Source: three-view drawing plus pictorial views. Frame: mm from the lowest corner of the part. A direction names the side the tool comes from. Give positions to 0.01 mm unless a question says otherwise; leave off trailing zeros. Loops run counter-clockwise (first coordinate to the right, second up) from the corner with the lowest first, then second, coordinate; pieces in that order, holes last. Notation, with made-up numbers: (74.25, 34) - (119.25, 34) arc R30 cw to (119.25, 73) - close; hole circle Ø9 at (73, 42.25). An arc over 180 degrees is marked (long way). Put each result on its own line as item: value.
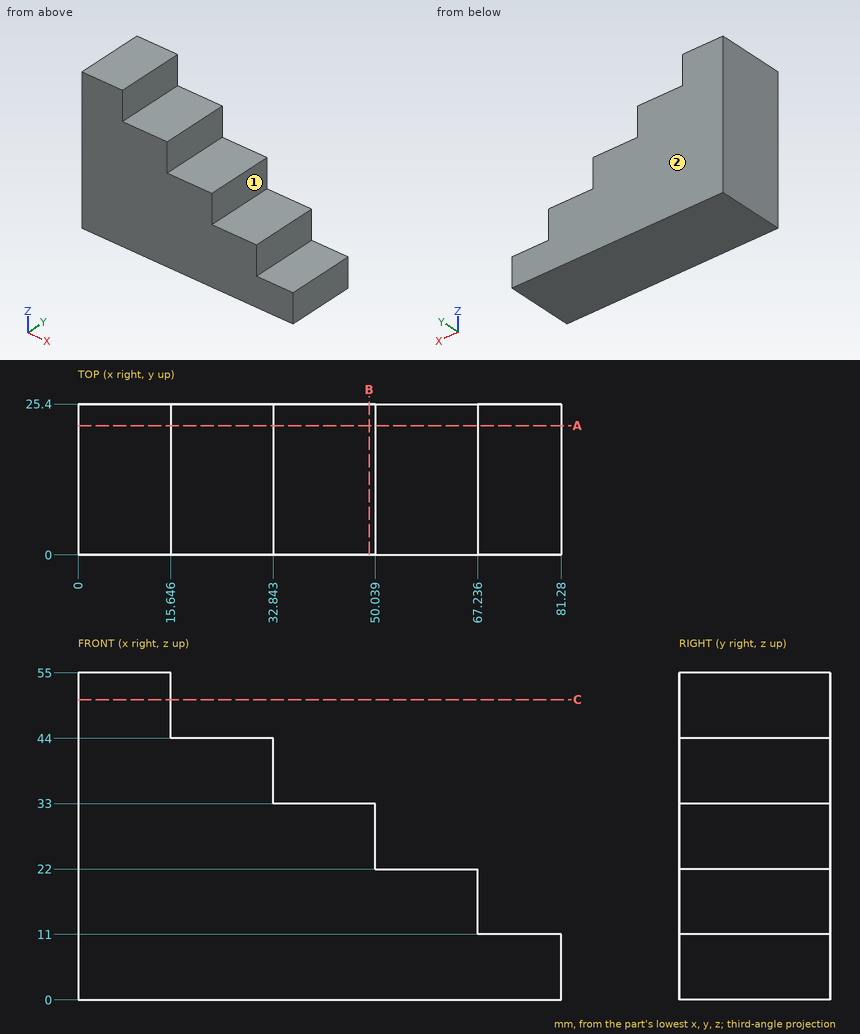
1) Section query A-A, the plane y = 21.75. Output: boundary loops of the cut face in (x, z).
Check result:
outline: (0, 0) - (81.28, 0) - (81.28, 11) - (67.24, 11) - (67.24, 22) - (50.04, 22) - (50.04, 33) - (32.84, 33) - (32.84, 44) - (15.65, 44) - (15.65, 55) - (0, 55) - close
2) Section query B-B, the plane x = 49. Output: boundary loops of the cut face in (y, z).
Check result:
outline: (0, 0) - (25.4, 0) - (25.4, 33) - (0, 33) - close
3) Section query C-C, the plane z = 50.5. Output: boundary loops of the cut face in (x, y).
Check result:
outline: (0, 0) - (15.65, 0) - (15.65, 25.4) - (0, 25.4) - close
4) Pin query (flat end, axial travel): P1, Ø6, axis at y = 8, z = 44, coming from the +X side; P2, Ø11, axis at x = 77.5, y = 12, coming from the +Z side; P3, Ø4, axis at x = 23, y = 14.5, coming from the +Z side. Return the tip coordinate at first contact, or that it passes through.
Check result:
P1: x = 32.84
P2: z = 11
P3: z = 44
5) Access query for the marked faces 1 and 2. Directions: +Z, -Z, +X, -X, +Y, -Y. A direction counts if a zero-diameter tool reaches every point of the face in a straight line with its end or side. Return the directions, or none.
Check result:
face 1: +Z, +X, +Y, -Y
face 2: +Z, -Z, +X, -X, +Y
6) Material intervals for line 1 along Z through (x, y) = (64, 3); line 2 along X through (y, z) = (21, 22.5); line 3 along X through (y, z) = (21.25, 20), sorted ascending. Write a range as [from, to].
Check result:
line 1: [0, 22]
line 2: [0, 50.04]
line 3: [0, 67.24]
